from build123d import *

# Parameters (mm, degrees)
SKETCH_R  = 8
PAD_DEPTH = 5


with BuildPart() as part:
    # Sketch → Pad (new body)
    with BuildSketch(Plane.XY):
        with BuildLine():
            ThreePointArc((-2.4, -9.707729), (10, 0), (-2.4, 9.707729))
            Line((-25.96, 3.883092), (-2.4, 9.707729))
            ThreePointArc((-25.96, 3.883092), (-29, 0), (-25.96, -3.883092))
            Line((-2.4, -9.707729), (-25.96, -3.883092))
        make_face()
        Circle(SKETCH_R, mode=Mode.SUBTRACT)
    extrude(amount=PAD_DEPTH)


solid = part.part
Read the model definition and answer for the solid it produces. Units are mm, in the model's axes. Give positions to 0.01 mm unless a question says otherwise; leave off trailing zeros. Write each loop counter-clockwise with the first axis right and the second up, starting at its lowest first coordinate (ties: lowest second). Pieces come first, ordered by that corner, then holes. Notation, with made-up numbers: (75.25, 66) - (91.25, 66) arc R33 cw to (91.25, 104) - close; hole circle Ø6 at (-33.5, -25). An arc over 180 degrees is marked (long way). Return JSON: item names as keys, results as strings.
Q1. Consider line 1 along Y through (x, z) = (0, 2.55); line 2 along Y through (x, z) = (-5, 0.65) (3 decimals); line 3 along X through (y, z) = (-1.5, 1.8). Determine where each line is inside the solid, lowest interval first. Write a range as [from, to].
Reply:
{"line 1": "[-10, -8], [8, 10]", "line 2": "[-9.065, -6.245], [6.245, 9.065]", "line 3": "[-28.71, -7.86], [7.86, 9.89]"}
Q2. A cutting plane is placed at A-A, the plane x = 0. Determine the outline of the cut face in (y, z).
Reply:
{"outline": "(-10, 0) - (-8, 0) - (-8, 5) - (-10, 5) - close; (8, 0) - (10, 0) - (10, 5) - (8, 5) - close"}
Q3. A cutting plane is placed at B-B, the plane y = 0. Determine the outline of the cut face in (x, z).
Reply:
{"outline": "(-29, 0) - (-8, 0) - (-8, 5) - (-29, 5) - close; (8, 0) - (10, 0) - (10, 5) - (8, 5) - close"}
Q4. A cutting plane is placed at D-D, the plane x = -25. Determine the outline of the cut face in (y, z).
Reply:
{"outline": "(-4.12, 0) - (4.12, 0) - (4.12, 5) - (-4.12, 5) - close"}
Q5. A cutting plane is placed at C-C, the plane z = 1.75. Determine the outline of the cut face in (x, y).
Reply:
{"outline": "(-25.96, -3.88) - (-2.4, -9.71) arc R10 ccw (long way) to (-2.4, 9.71) - (-25.96, 3.88) arc R4 ccw to start; hole circle Ø16 at (0, 0)"}
Q6. For a pull along X with two mould halves and no side action, classify faces 1 (the face through (-1.73, -7.81, 2.46)), 2 (the face through (-14.015, -6.836, 2.465)), 3 (the face through (10, 0, 2)), 4 (the face through (-14, 0, 0)) as released by +X, released by -X, zero draft, split by the parting line, or undercut.
Reply:
{"face 1": "undercut", "face 2": "released by -X", "face 3": "split by the parting line", "face 4": "zero draft"}
